Check sheet for the modelled part. Datum: model origin and axes. Units: mm. Coordinates: 2 decimals unless noted, no trailing zeros. Loops run counter-clockwise (first coordinate to the right, second up) from the corner with the lowest first, then second, coordinate; pieces in that order, holes last. Notation, with made-up numbers: (-2, 89.5) -> (23, 89.5) arc R11 ccw to (23, 102.5) -> close; hole circle Ø8 at (16, -7.5). An arc over 180 degrees is marked (long way). Use one line per item in the form item = value.
from build123d import *

# Parameters (mm, degrees)
SKETCH1_R                      = 3.5
BOSS_EXTRUDE1_DEPTH            = 0.75
F_3_2_3_2_DIAMETER_HOLE1_D     = 3.2
F_3_2_3_2_DIAMETER_HOLE1_DEPTH = 10
F_3_2_3_2_DIAMETER_HOLE1_TIP   = 0.96137699
CUT_EXTRUDE1_DEPTH             = 123.2407972
FILLET1_R                      = 2
SKETCH7_R                      = 9.5
CUT_EXTRUDE2_DEPTH             = 123.240797318


with BuildPart() as part:
    # Sketch1 → Boss-Extrude1 (new, symmetric)
    with BuildSketch(Plane(origin=(0, 0, 0), x_dir=(1, 0, 0), z_dir=(0, 1, 0))):
        with BuildLine():
            ThreePointArc((-37.239092363, -21.5), (-43, 0), (-37.239092363, 21.5))
            ThreePointArc((-37.239092363, 21.5), (-36.658838331, 22.248681329), (-35.899079455, 22.81435343))
            ThreePointArc((-35.899079455, 22.81435343), (-70.492179883, 10.7556392), (-107.126701642, 10.839315166))
            ThreePointArc((-107.126701642, 10.839315166), (-120, 0), (-107.126701642, -10.839315166))
            ThreePointArc((-107.126701642, -10.839315166), (-70.492179883, -10.7556392), (-35.899079455, -22.81435343))
            ThreePointArc((-35.899079455, -22.81435343), (-36.658838331, -22.248681329), (-37.239092363, -21.5))
        make_face()
        with BuildLine():
            ThreePointArc((-31.176914536, 18), (-35.958003449, 16.718911087), (-37.239092363, 21.5))
            ThreePointArc((-37.239092363, 21.5), (-43, 0), (-37.239092363, -21.5))
            ThreePointArc((-37.239092363, -21.5), (-35.958003449, -16.718911087), (-31.176914536, -18))
            ThreePointArc((-31.176914536, -18), (-36, 0), (-31.176914536, 18))
        make_face()
        with Locations((-34.208003449, -19.75)):
            Circle(SKETCH1_R)
        with Locations((-34.208003449, 19.75)):
            Circle(SKETCH1_R)
    extrude(amount=BOSS_EXTRUDE1_DEPTH, both=True)

    # Ø3.2 (3.2) Diameter Hole1
    with Locations(Plane(origin=(0, 0.75, 0), x_dir=(1, 0, 0), z_dir=(0, 1, 0))):
        with Locations((-34.208003449, 19.75), (-34.208003449, -19.75), (-95.790276336, 5.979398024), (-95.790276336, -5.979398024)):
            Hole(F_3_2_3_2_DIAMETER_HOLE1_D / 2, depth=F_3_2_3_2_DIAMETER_HOLE1_DEPTH)
            with Locations((0, 0, -(F_3_2_3_2_DIAMETER_HOLE1_DEPTH + F_3_2_3_2_DIAMETER_HOLE1_TIP / 2))):  # 118° drill point
                Cone(0, F_3_2_3_2_DIAMETER_HOLE1_D / 2, F_3_2_3_2_DIAMETER_HOLE1_TIP, mode=Mode.SUBTRACT)

    # Sketch6 → Cut-Extrude1 (cut, through all)
    with BuildSketch(Plane(origin=(0, 0.75, 0), x_dir=(1, 0, 0), z_dir=(0, 1, 0))):
        with BuildLine():
            Line((-72.469338063, -3.369046694), (-49.802019621, 0))
            Line((-49.802019621, 0), (-72.469338063, 3.369046694))
            ThreePointArc((-72.469338063, 3.369046694), (-85.377857375, 2.290839769), (-98.326107181, 2.65857332))
            ThreePointArc((-98.326107181, 2.65857332), (-98, 0), (-98.326107181, -2.65857332))
            ThreePointArc((-98.326107181, -2.65857332), (-85.377857375, -2.290839769), (-72.469338063, -3.369046694))
        make_face()
        with BuildLine():
            Line((-66.096117167, 4.443764231), (-42.988154947, 1.009224591))
            ThreePointArc((-42.988154947, 1.009224591), (-42.467311238, 6.747405149), (-41.183985346, 12.36443897))
            ThreePointArc((-41.183985346, 12.36443897), (-53.416219701, 7.70010587), (-66.096117167, 4.443764231))
        make_face()
        with BuildLine():
            ThreePointArc((-41.183985346, -12.36443897), (-42.467311238, -6.747405149), (-42.988154947, -1.009224591))
            Line((-42.988154947, -1.009224591), (-66.096117167, -4.443764231))
            ThreePointArc((-66.096117167, -4.443764231), (-53.416219701, -7.70010587), (-41.183985346, -12.36443897))
        make_face()
    extrude(amount=-CUT_EXTRUDE1_DEPTH, mode=Mode.SUBTRACT)

    # Fillet1
    fillet1_edges = [part.edges().sort_by_distance(p)[0] for p in [
        (-98.326107181, 0, 2.65857332),
        (-98.326107181, 0, -2.65857332),
        (-72.469338063, 0, -3.369046694),
        (-49.802019621, 0, 0),
        (-72.469338063, 0, 3.369046694),
        (-41.183985346, 0, -12.36443897),
        (-42.988154947, 0, -1.009224591),
        (-66.096117167, 0, -4.443764231),
        (-42.988154947, 0, 1.009224591),
        (-41.183985346, 0, 12.36443897),
        (-66.096117167, 0, 4.443764231),
    ]]
    fillet(fillet1_edges, radius=FILLET1_R)

    # Sketch7 → Cut-Extrude2 (cut, through all)
    with BuildSketch(Plane(origin=(0, 0.75, 0), x_dir=(1, 0, 0), z_dir=(0, 1, 0))):
        with Locations(Location((-109, 0, 0), (0, 0, 270))):
            Circle(SKETCH7_R)
    extrude(amount=-CUT_EXTRUDE2_DEPTH, mode=Mode.SUBTRACT)


solid = part.part
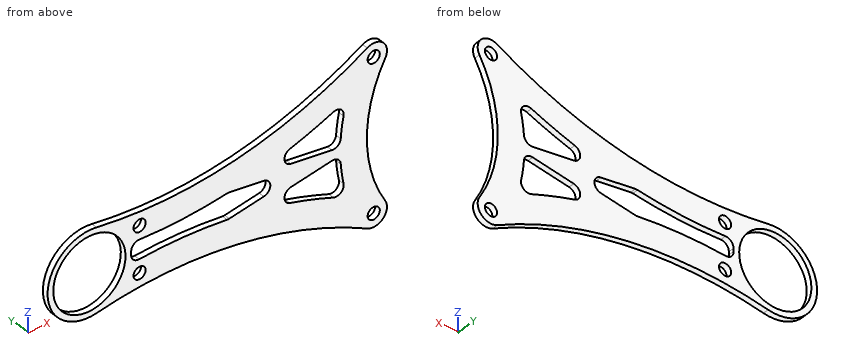
(1) Section check B-B, the plane z = -19.75. Record the boundary of the cut face in (x, y), plus the area to 3 significant figures.
Established:
outline = (-41.88, -0.75) -> (-35.81, -0.75) -> (-35.81, 0.75) -> (-41.88, 0.75) -> close; (-32.61, -0.75) -> (-30.71, -0.75) -> (-30.71, 0.75) -> (-32.61, 0.75) -> close
area = 12.0 mm²
(2) Section check D-D, the plane y = -0.25. Give the number of separate pieces and of enclosed holes in the cut face, plus the area to 3 significant figures.
Established:
separate_pieces = 1
enclosed_holes = 8
area = 1,440 mm²
(3) Section check A-A, the plane x = -109. Record the boundary of the cut face in (y, z).
Established:
outline = (-0.75, -11) -> (0.75, -11) -> (0.75, -9.5) -> (-0.75, -9.5) -> close; (-0.75, 9.5) -> (0.75, 9.5) -> (0.75, 11) -> (-0.75, 11) -> close
(4) Scan lines: line 1 along X through (y, z) = (0.2, 0); line 2 along Z through (x, y) = (-81.5, -0.2); line 3 along X through (y, z) = (-0.35, -0.5). Record each from-to range of solid material in increasing order.
Established:
line_1 = -120 to -118.5, -99.5 to -98, -61.41 to -36
line_2 = -9.48 to -2.46, 2.46 to 9.48
line_3 = -119.99 to -118.49, -99.51 to -98.01, -61.47 to -36
(5) Section check C-C, the plane x = -54.5. Record the boundary of the cut face in (y, z), plus the area to 3 significant figures.
Established:
outline = (-0.75, -14.71) -> (0.75, -14.71) -> (0.75, -7.36) -> (-0.75, -7.36) -> close; (-0.75, -2.72) -> (0.75, -2.72) -> (0.75, 2.72) -> (-0.75, 2.72) -> close; (-0.75, 7.36) -> (0.75, 7.36) -> (0.75, 14.71) -> (-0.75, 14.71) -> close
area = 30.2 mm²
